Answer from the drawing. Dimensions are ordinates in mm from the lowest x, y and z of the part. A direction names the side the tool comes from. Coordinates: 2 decimals unless noted, no trailing zeros. Order: outer loops, then holes, each group sorted by start corner. A loop starts at its lowest first (then second) coordinate and runs counter-clockwise, first axis right, second up. Notation, with made-up numbers: (21.25, -10.75) -> (42.25, -10.75) arc R10 ccw to (42.25, -2.75) -> close; hole circle Ø2 at (-29, 32). An arc over 180 degrees is marked (long way). Answer in a Markdown table with one row per item.
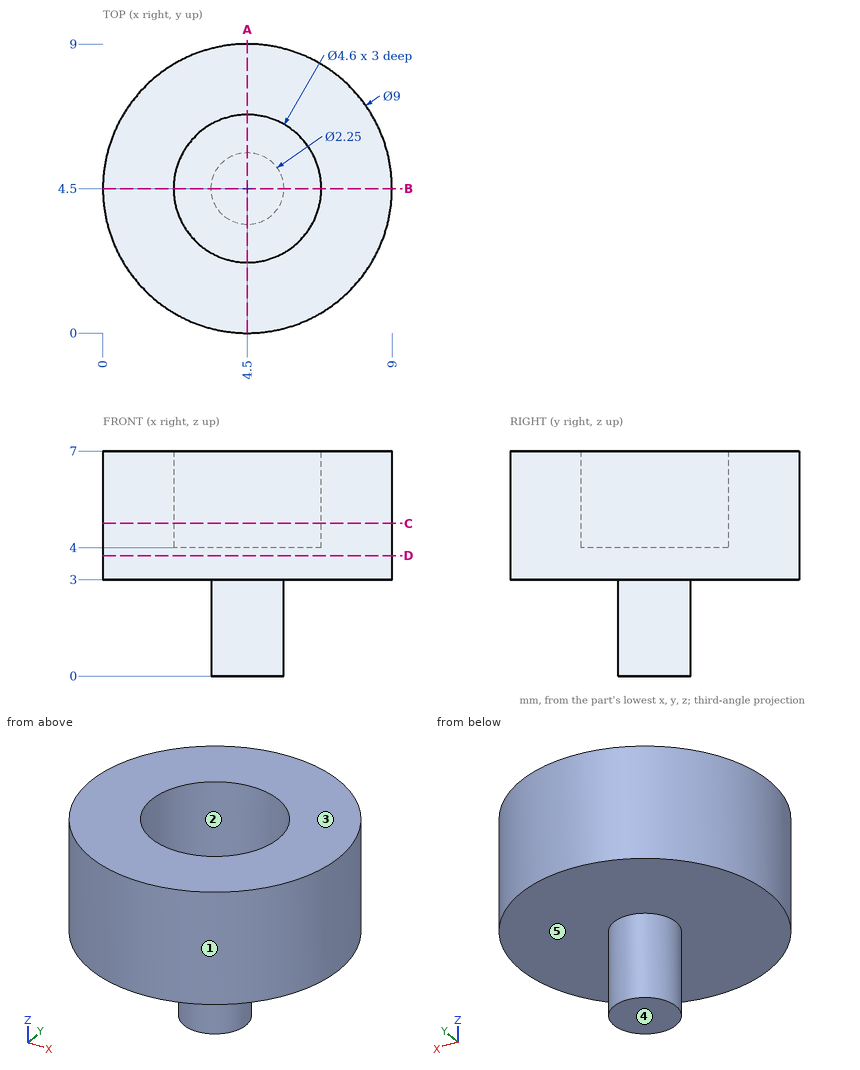
(1) A cutting plane is placed at A-A, the plane x = 4.5. Determine the outline of the cut face in (y, z) (3 decimals).
Check values:
| item | result |
|---|---|
| outline | (0, 3) -> (3.375, 3) -> (3.375, 0) -> (5.625, 0) -> (5.625, 3) -> (9, 3) -> (9, 7) -> (6.8, 7) -> (6.8, 4) -> (2.2, 4) -> (2.2, 7) -> (0, 7) -> close |
(2) Which of the six approach directions +Z, -Z, +X, -X, +Y, -Y give full straight-line access (tool end or side, diameter ignored) to the marked faces 4 and 5?
Check values:
| item | result |
|---|---|
| face 4 | -Z, +X, -X, +Y, -Y |
| face 5 | -Z |
(3) A cutting plane is placed at C-C, the plane z = 4.75. Determine the outline of the cut face in (x, y), then the cut area to 3 significant figures.
Check values:
| item | result |
|---|---|
| outline | circle Ø9 at (4.5, 4.5); hole circle Ø4.6 at (4.5, 4.5) |
| area | 47.0 mm² |
(4) For a pull along Y with two mould halves and no side action, classify the marked faces 1, 2 and 3 as released by +Y, released by -Y, zero draft, split by the parting line, or undercut.
Check values:
| item | result |
|---|---|
| face 1 | split by the parting line |
| face 2 | undercut |
| face 3 | zero draft |
(5) Find the intervals of material crossed by line 1 along Y through (x, z) = (4.5, 5.4); line 2 along Z through (x, y) = (3.5, 4.75); line 3 along Z through (x, y) = (8.5, 2.5), in increasing order. Write a range as from..to.
Check values:
| item | result |
|---|---|
| line 1 | 0..2.2, 6.8..9 |
| line 2 | 0..4 |
| line 3 | 3..7 |
(6) Flat-ended cylindrical pins translate along their axes: pin 1 (1.5 mm diameter, centred on x = 7.5, z = 4.5, fed in from -Y); pin 2 (1 mm diameter, centred on y = 1, z = 5, fed in from -X); pin 3 (1.5 mm diameter, centred on y = 2.5, z = 4, fed in from -X). Find the tip coordinate at first contact, or state that the pin passes through.
Check values:
| item | result |
|---|---|
| pin 1 | y = 0.6 |
| pin 2 | x = 1.15 |
| pin 3 | x = 0.18 |
(7) A cutting plane is placed at D-D, the plane z = 3.75. Determine the outline of the cut face in (x, y), then the cut area to 3 significant figures.
Check values:
| item | result |
|---|---|
| outline | circle Ø9 at (4.5, 4.5) |
| area | 63.6 mm² |
